Can you work these out from the model? Positions are in its coordinate system, mm. Round coordinates to 2 decimals unless told otherwise and drop trailing zeros. Loops run counter-clockwise (first coordinate to the right, second up) from the corner with the lowest first, then second, coordinate; pieces in that order, holes last. Notation, with made-up numbers: M -25,28 L -10,28 A21 ccw -10,45 Z; hole C 78.25,43.5 d5. An arc over 180 degrees is marked long. Answer as CSV lines item,"result".
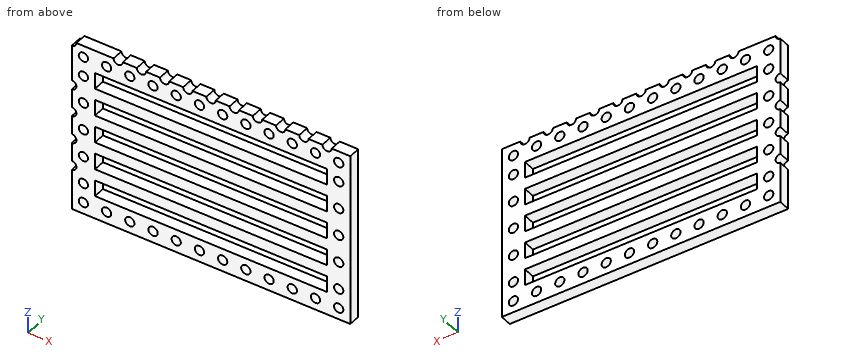
Autodesk Inventor part; units mm, degrees
ref_plane "YZ Plane" through (0, 0, 0) normal (1, 0, 0) x (0, 1, 0)
ref_plane "XZ Plane" through (0, 0, 0) normal (0, 1, 0) x (-1, 0, 0)
ref_plane "XY Plane" through (0, 0, 0) normal (0, 0, 1) x (1, 0, 0)
sketch "Sketch1" plane through (0, 0, 0) normal (0, 1, 0) x (-1, 0, 0)
  line L0 (0, 0) -> (60, 0)
  line L1 (60, 0) -> (60, -37.5)
  line L2 (60, -37.5) -> (0, -37.5)
  line L3 (0, -37.5) -> (0, 0)
  line L4 (60, 0) -> (55, 0)
  line L5 (55, 0) -> (55, -5)
  line L6 (55, -5) -> (60, -5)
  line L7 (60, -5) -> (60, 0)
  line L8 (0, -37.5) -> (5, -37.5)
  line L9 (5, -37.5) -> (5, -32.5)
  line L10 (5, -32.5) -> (0, -32.5)
  line L11 (0, -32.5) -> (0, -37.5)
  line L12 (55, -5) -> (5, -5)
  line L13 (5, -5) -> (5, -32.5)
  line L14 (5, -32.5) -> (55, -32.5)
  line L15 (55, -32.5) -> (55, -5)
  line L16 (5, -5) -> (5, -8.5)
  line L17 (5, -8.5) -> (5, -11)
  line L18 (5, -11) -> (5, -14.5)
  line L19 (5, -14.5) -> (5, -17)
  line L20 (5, -17) -> (5, -20.5)
  line L21 (5, -20.5) -> (5, -23)
  line L22 (5, -23) -> (5, -26.5)
  line L23 (5, -26.5) -> (5, -29)
  line L24 (5, -29) -> (5, -32.5)
  line L25 (5, -8.5) -> (55, -8.5)
  line L26 (55, -8.5) -> (55, -11)
  line L27 (55, -11) -> (5, -11)
  line L28 (5, -11) -> (5, -8.5)
  line L29 (5, -14.5) -> (55, -14.5)
  line L30 (55, -14.5) -> (55, -17)
  line L31 (55, -17) -> (5, -17)
  line L32 (5, -17) -> (5, -14.5)
  line L33 (5, -20.5) -> (55, -20.5)
  line L34 (55, -20.5) -> (55, -23)
  line L35 (55, -23) -> (5, -23)
  line L36 (5, -23) -> (5, -20.5)
  line L37 (5, -26.5) -> (55, -26.5)
  line L38 (55, -26.5) -> (55, -29)
  line L39 (55, -29) -> (5, -29)
  line L40 (5, -29) -> (5, -26.5)
  line L41 (0, 0) -> (2.5, 0)
  line L42 (2.5, 0) -> (2.5, -2.5)
  line L43 (2.5, -2.5) -> (0, -2.5)
  line L44 (0, -2.5) -> (0, 0)
  circle A0 centre (2.5, -2.5) radius 1
  line L45 (5, -6.75) -> (2.5, -6.75)
  line L46 (5, -12.75) -> (2.5, -12.75)
  line L47 (5, -18.75) -> (2.5, -18.75)
  line L48 (5, -24.75) -> (2.5, -24.75)
  line L49 (5, -30.75) -> (2.5, -30.75)
  line L50 (5, -35) -> (2.5, -35)
  circle A1 centre (2.5, -35) radius 1
  circle A2 centre (2.5, -30.75) radius 1
  circle A3 centre (2.5, -24.75) radius 1
  circle A4 centre (2.5, -18.75) radius 1
  circle A5 centre (2.5, -12.75) radius 1
  circle A6 centre (2.5, -6.75) radius 1
  line L51 (60, 0) -> (57.5, 0)
  line L52 (57.5, 0) -> (57.5, -2.5)
  line L53 (57.5, -2.5) -> (60, -2.5)
  line L54 (60, -2.5) -> (60, 0)
  circle A7 centre (57.5, -2.5) radius 1
  circle A8 centre (57.5, -6.75) radius 1
  circle A9 centre (57.5, -12.75) radius 1
  circle A10 centre (57.5, -18.75) radius 1
  circle A11 centre (57.5, -24.75) radius 1
  circle A12 centre (57.5, -30.75) radius 1
  circle A13 centre (57.5, -35) radius 1
  line L55 (57.5, -35) -> (52.5, -35)
  line L56 (52.5, -35) -> (47.5, -35)
  line L57 (47.5, -35) -> (42.5, -35)
  line L58 (42.5, -35) -> (37.5, -35)
  line L59 (37.5, -35) -> (32.5, -35)
  line L60 (32.5, -35) -> (27.5, -35)
  line L61 (27.5, -35) -> (22.5, -35)
  line L62 (22.5, -35) -> (17.5, -35)
  line L63 (17.5, -35) -> (12.5, -35)
  line L64 (12.5, -35) -> (7.5, -35)
  circle A14 centre (52.5, -35) radius 1
  circle A15 centre (47.5, -35) radius 1
  circle A16 centre (42.5, -35) radius 1
  circle A17 centre (37.5, -35) radius 1
  circle A18 centre (32.5, -35) radius 1
  circle A19 centre (27.5, -35) radius 1
  circle A20 centre (22.5, -35) radius 1
  circle A21 centre (17.5, -35) radius 1
  circle A22 centre (12.5, -35) radius 1
  circle A23 centre (7.5, -35) radius 1
  circle A24 centre (52.5, -2.5) radius 1
  circle A25 centre (47.5, -2.5) radius 1
  circle A26 centre (42.5, -2.5) radius 1
  circle A27 centre (37.5, -2.5) radius 1
  circle A28 centre (32.5, -2.5) radius 1
  circle A29 centre (27.5, -2.5) radius 1
  circle A30 centre (22.5, -2.5) radius 1
  circle A31 centre (17.5, -2.5) radius 1
  circle A32 centre (12.5, -2.5) radius 1
  circle A33 centre (7.5, -2.5) radius 1
  line L65 (0, 0) -> (5, 0)
  line L66 (5, 0) -> (10, 0)
  line L67 (10, 0) -> (15, 0)
  line L68 (15, 0) -> (20, 0)
  line L69 (20, 0) -> (25, 0)
  line L70 (25, 0) -> (30, 0)
  line L71 (30, 0) -> (35, 0)
  line L72 (35, 0) -> (40, 0)
  line L73 (40, 0) -> (45, 0)
  line L74 (45, 0) -> (50, 0)
  line L75 (50, 0) -> (55, 0)
  circle A34 centre (5, 0) radius 1
  circle A35 centre (10, 0) radius 1
  circle A36 centre (15, 0) radius 1
  circle A37 centre (20, 0) radius 1
  circle A38 centre (25, 0) radius 1
  circle A39 centre (30, 0) radius 1
  circle A40 centre (35, 0) radius 1
  circle A41 centre (40, 0) radius 1
  circle A42 centre (45, 0) radius 1
  circle A43 centre (50, 0) radius 1
  circle A44 centre (60, 0) radius 1
  line L76 (55, -9.75) -> (60, -9.75)
  line L77 (55, -15.75) -> (60, -15.75)
  line L78 (55, -21.75) -> (60, -21.75)
  line L79 (55, -27.75) -> (60, -27.75)
  circle A45 centre (60, -27.75) radius 1
  circle A46 centre (60, -21.75) radius 1
  circle A47 centre (60, -15.75) radius 1
  circle A48 centre (60, -9.75) radius 1
  point P0 (60, -1)
  point P1 (59, 0)
  point P2 (51, 0)
  point P3 (49, 0)
  point P4 (46, 0)
  point P5 (44, 0)
  point P6 (41, 0)
  point P7 (39, 0)
  point P8 (36, 0)
  point P9 (34, 0)
  point P10 (31, 0)
  point P11 (29, 0)
  point P12 (26, 0)
  point P13 (24, 0)
  point P14 (21, 0)
  point P15 (19, 0)
  point P16 (16, 0)
  point P17 (14, 0)
  point P18 (11, 0)
  point P19 (9, 0)
  point P20 (6, 0)
  point P21 (4, 0)
  point P22 (60, -28.75)
  point P23 (60, -26.75)
  point P24 (60, -22.75)
  point P25 (60, -20.75)
  point P26 (60, -16.75)
  point P27 (60, -14.75)
  point P28 (60, -10.75)
  point P29 (60, -8.75)
  dimension "d0" = 60
  dimension "d1" = 37.5
  dimension "d2" = 5
  dimension "d3" = 5
  dimension "d4" = 5
  dimension "d5" = 5
  dimension "d6" = 3.5
  dimension "d7" = 2.5
  dimension "d8" = 3.5
  dimension "d9" = 2.5
  dimension "d10" = 3.5
  dimension "d11" = 2.5
  dimension "d12" = 3.5
  dimension "d13" = 2.5
  dimension "d14" = 3.5
  dimension "d15" = 2.5
  dimension "d16" = 2.5
  dimension "d17" = 2
  dimension "d18" = 2
  dimension "d19" = 2
  dimension "d20" = 2
  dimension "d21" = 2
  dimension "d22" = 2
  dimension "d23" = 2
  dimension "d24" = 2.5
  dimension "d25" = 2.5
  dimension "d26" = 2
  dimension "d27" = 2
  dimension "d28" = 2
  dimension "d29" = 2
  dimension "d30" = 2
  dimension "d31" = 2
  dimension "d32" = 2
  dimension "d33" = 5
  dimension "d34" = 5
  dimension "d35" = 5
  dimension "d36" = 5
  dimension "d37" = 5
  dimension "d38" = 5
  dimension "d39" = 5
  dimension "d40" = 5
  dimension "d41" = 5
  dimension "d42" = 5
  dimension "d43" = 2
  dimension "d44" = 2
  dimension "d45" = 2
  dimension "d46" = 2
  dimension "d47" = 2
  dimension "d48" = 2
  dimension "d49" = 2
  dimension "d50" = 2
  dimension "d51" = 2
  dimension "d52" = 2
  dimension "d53" = 2
  dimension "d54" = 2
  dimension "d55" = 2
  dimension "d56" = 2
  dimension "d57" = 2
  dimension "d58" = 2
  dimension "d59" = 2
  dimension "d60" = 2
  dimension "d61" = 2
  dimension "d62" = 2
  dimension "d63" = 5
extrude "Extrusion1" add sketch "Sketch1" along normal blind 2.5 contours L0 L42 A0 L43 L3 | L0 A34 A35 A36 A37 A38 A39 A40 A41 A42 A43 L5 L12 L13 L10 L3 L43 A0 L42 | L10 L9 L2 L3 | L14 L15 L79 A45 L1 L2 L9 | L13 L37 L15 L39 | L15 L78 A46 L1 A45 L79 | L13 L33 L15 L35 | L15 L77 A47 L1 A46 L78 | L13 L29 L15 L31 | L15 L76 A48 L1 A47 L77 | L13 L25 L15 L27 | L15 L6 L1 A48 L76 | L5 L0 L52 A7 L53 L1 L6 | L53 A7 L52 L0 A44 L1
properties part number "placa_galbena"
Item 1: If we section it at A-A on x = -42.5: State how many separate pieces and enclosed holes the cut face has, then the cut area to 3 significant figures.
Output:
separate pieces,"8"
enclosed holes,"0"
area,"40.0 mm2"
Item 2: If I drill on line 1 along X through (y, z) = (0.95, -29.5); line 2 along Z through (x, y) = (-10.5, 0.25); line 3 along X through (y, z) = (2.25, -19.5), over which ranges is the centre line in solid material (lowest first)? Write a range as from..to.
Output:
line 1,"x = -60..-55, -5..0"
line 2,"z = -37.5..-32.5, -29..-26.5, -23..-20.5, -17..-14.5, -11..-8.5, -5..-0.87"
line 3,"x = -60..-58.16, -56.84..-55, -5..-3.16, -1.84..0"
Item 3: If we section it at C-C on x = -35: Write out the boundary of the cut face in (y, z).
Output:
outline,"M 0,-37.5 L 2.5,-37.5 L 2.5,-32.5 L 0,-32.5 Z; M 0,-29 L 2.5,-29 L 2.5,-26.5 L 0,-26.5 Z; M 0,-23 L 2.5,-23 L 2.5,-20.5 L 0,-20.5 Z; M 0,-17 L 2.5,-17 L 2.5,-14.5 L 0,-14.5 Z; M 0,-11 L 2.5,-11 L 2.5,-8.5 L 0,-8.5 Z; M 0,-5 L 2.5,-5 L 2.5,-1 L 0,-1 Z"
Item 4: If we section it at B-B on z = -18.75: Write out the boundary of the cut face in (x, y), then the cut area to 3 significant figures.
Output:
outline,"M -60,0 L -58.5,0 L -58.5,2.5 L -60,2.5 Z; M -56.5,0 L -55,0 L -55,2.5 L -56.5,2.5 Z; M -5,0 L -3.5,0 L -3.5,2.5 L -5,2.5 Z; M -1.5,0 L 0,0 L 0,2.5 L -1.5,2.5 Z"
area,"15.0 mm2"
